Source: three-view drawing plus pictorial views. Frame: mm from the lowest corner of the part. Give positions to 0.01 mm unless a question says otherwise; leave off trailing zeros. Loops run counter-clockwise (first coordinate to the right, second up) from the corner with the lowest first, then second, coordinate; pieces in that order, holes last. Notation, with made-up numbers: (6.5, -37.5) -> (12.5, -37.5) arc R23 ccw to (12.5, -6.5) -> close; hole circle Ø2 at (-0.75, 5.25). An arc over 180 degrees is marked (long way). Answer as a JSON object with one key per item and string values. Group by question number.
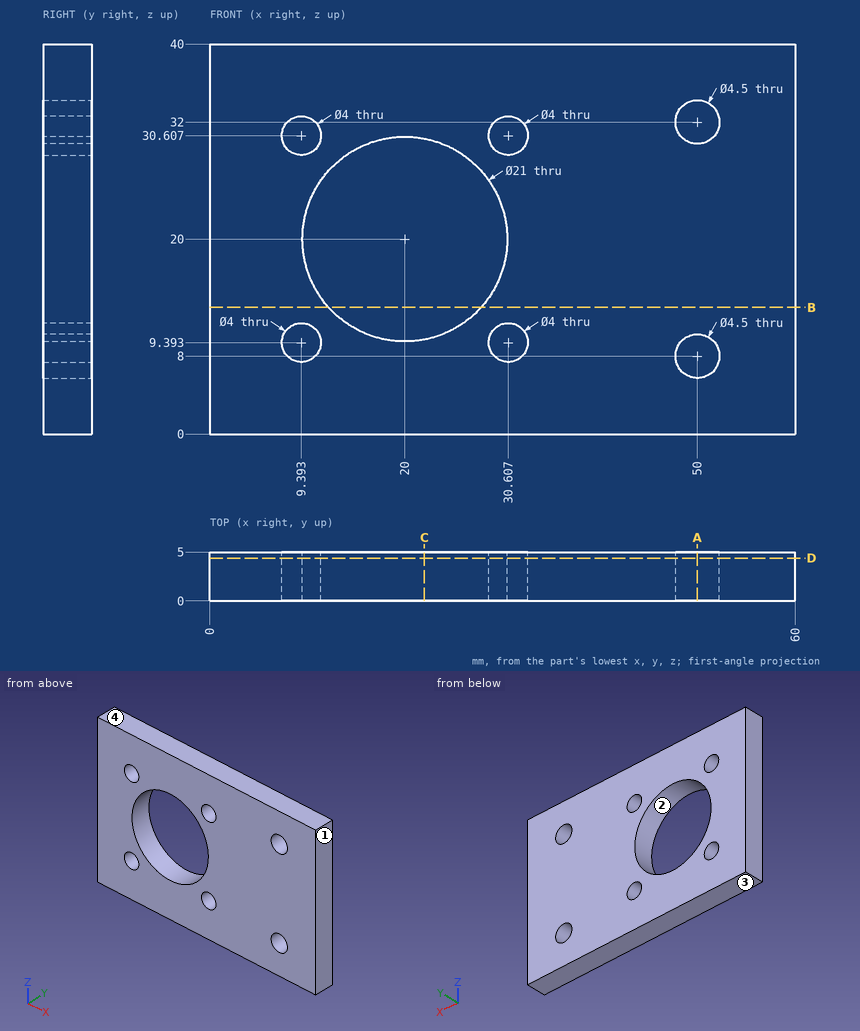
Q1. Ray query, probe 1 along X at (y, z) = (3.05, 8); probe 2 along Z at (x, y) = (29.5, 1.1) (1 decimal); probe 3 along X at (y, z) = (1.65, 24.5) (1 decimal). Return the intervals inside material, ascending.
Q2. Pin query (flat end, axial travel): pin 1 Ø3.5 at (x, z) = (9.39, 9.39) entering from +Y. Return the tip coordinate at first contact, or that it passes through.
Q3. Section D-D on y = 4.4. Return the cut outline in (x, z).
Q4. Section B-B on z = 13. Return the cut outline in (x, y).
Q5. Section C-C on x = 22. Return the cut outline in (y, z).
Q6. Pull-direction query (Z, two-part tool) for the marked faces 1, 2, 3 and 4; classes: +Z half, -Z half, draft (parallel to the pull), parting line (faces both ways), or undercut.
Q7. Section A-A on x = 50. Return the cut outline in (y, z).
Numbers:
{
 "1": {"probe 1": "x = 0 to 7.96, 10.83 to 29.17, 32.04 to 47.75, 52.25 to 60", "probe 2": "z = 0 to 7.7, 11.1 to 15.5, 24.5 to 28.9, 32.3 to 40", "probe 3": "x = 0 to 10.5, 29.5 to 60"},
 "2": {"pin 1": "passes through"},
 "3": {"outline": "(0, 0) -> (60, 0) -> (60, 40) -> (0, 40) -> close; hole circle Ø4 at (9.39, 9.39); hole circle Ø4 at (9.39, 30.61); hole circle Ø21 at (20, 20); hole circle Ø4 at (30.61, 9.39); hole circle Ø4 at (30.61, 30.61); hole circle Ø4.5 at (50, 8); hole circle Ø4.5 at (50, 32)"},
 "4": {"outline": "(0, 0) -> (12.17, 0) -> (12.17, 5) -> (0, 5) -> close; (27.83, 0) -> (60, 0) -> (60, 5) -> (27.83, 5) -> close"},
 "5": {"outline": "(0, 0) -> (5, 0) -> (5, 9.69) -> (0, 9.69) -> close; (0, 30.31) -> (5, 30.31) -> (5, 40) -> (0, 40) -> close"},
 "6": {"face 1": "draft", "face 2": "undercut", "face 3": "-Z half", "face 4": "+Z half"},
 "7": {"outline": "(0, 0) -> (5, 0) -> (5, 5.75) -> (0, 5.75) -> close; (0, 10.25) -> (5, 10.25) -> (5, 29.75) -> (0, 29.75) -> close; (0, 34.25) -> (5, 34.25) -> (5, 40) -> (0, 40) -> close"}
}
